Geometry check sheet. Reference: drawing and pictorial views, mm from the part's lowest x, y, z. Give positions to 0.01 mm unless a question says otherwise; leave off trailing zeros. Loops run counter-clockwise (first coordinate to the right, second up) from the corner with the lowest first, then second, coordinate; pieces in that order, holes last. Notation, with made-up numbers: (75, -4) - (100, -4) arc R20 cw to (100, 29) - close; hole circle Ø2 at (-36.5, 26). An arc over 180 degrees is marked (long way). Put each result on its own line as item: value. Start each with the question number.
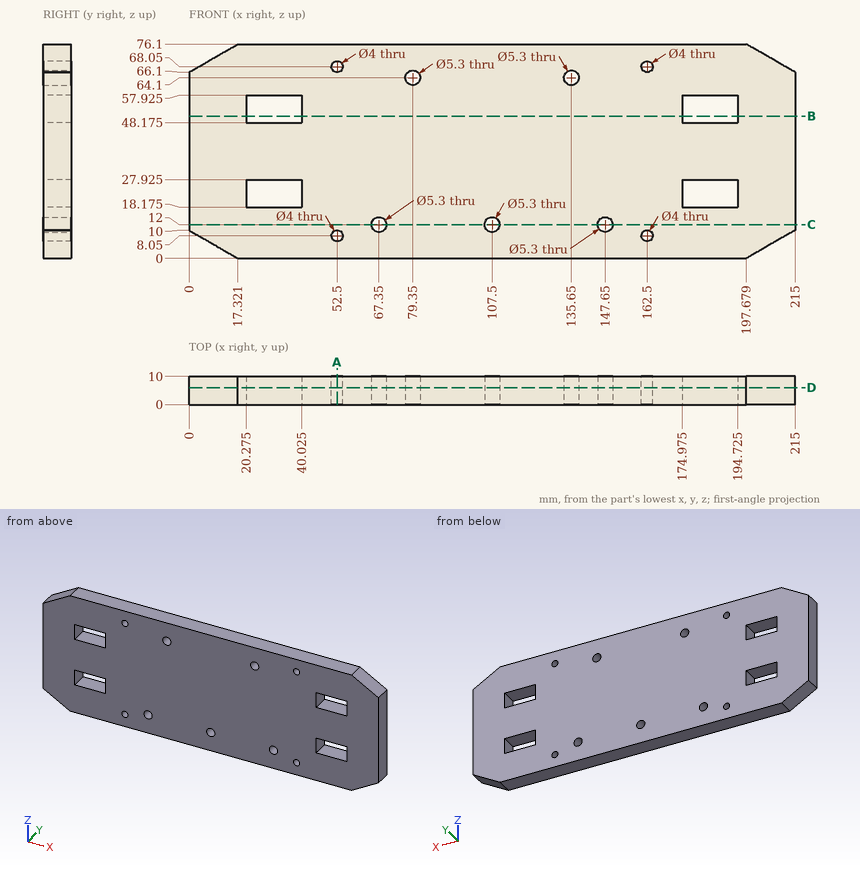
1) Scan lines: line 1 along Z through (x, y) = (181, 4) (1 decimal); line 2 along Z through (x, y) = (52.5, 5.75); line 3 along X through (y, z) = (4.5, 12). Record each from-to range of solid material in increasing order. Write a range as from..to.
2) Section check C-C, the plane z = 12. Enter the section's corners in (x, y).
3) Depth check by flat-ended pin: P1, Ø2.5, axis at x = 162.5, z = 68.05, coming from the +Y side. Enter the tip coordinate at first touch or a pass-through.
4) Section check A-A, the plane x = 52.5. Enter the section's corners in (y, z).
5) Section check D-D, the plane y = 6. State how many separate pieces and enclosed holes the cut face has, plus the area to 3 significant figures.
6) Section check B-B, the plane z = 50.5. Enter the section's corners in (x, y) (1 decimal).
Results are:
1. line 1: z = 0..18.2, 27.9..48.2, 57.9..76.1
1. line 2: z = 0..6.05, 10.05..66.05, 70.05..76.1
1. line 3: x = 0..64.7, 70..104.85, 110.15..145, 150.3..215
2. outline: (0, 0) - (64.7, 0) - (64.7, 10) - (0, 10) - close; (70, 0) - (104.85, 0) - (104.85, 10) - (70, 10) - close; (110.15, 0) - (145, 0) - (145, 10) - (110.15, 10) - close; (150.3, 0) - (215, 0) - (215, 10) - (150.3, 10) - close
3. P1: passes through
4. outline: (0, 0) - (10, 0) - (10, 6.05) - (0, 6.05) - close; (0, 10.05) - (10, 10.05) - (10, 66.05) - (0, 66.05) - close; (0, 70.05) - (10, 70.05) - (10, 76.1) - (0, 76.1) - close
5. separate pieces: 1
5. enclosed holes: 13
5. area: 15,100 mm2
6. outline: (0, 0) - (20.3, 0) - (20.3, 10) - (0, 10) - close; (40, 0) - (175, 0) - (175, 10) - (40, 10) - close; (194.7, 0) - (215, 0) - (215, 10) - (194.7, 10) - close
